Could you check a few things on this model? Use its own coordinates, in mm. A direction names the side the tool comes from. Give positions to 0.01 mm unless a question says otherwise; leave off trailing zeros. Write each loop counter-clockwise with the first axis right and the second up, starting at its lowest first coordinate (ties: lowest second). Pieces come first, ordered by that corner, then holes. Notation, with made-up numbers: (-20, 50) - (10, 50) arc R34 cw to (10, 85) - close; hole circle Ø9 at (84, 48). An arc over 180 degrees is marked (long way). Answer in a Markdown table with one row per item.
from build123d import *

# Parameters (mm, degrees)
SKETCH_1_R          = 1
SKETCH_1_R_2        = 1.5
EXTRUDE_1_DEPTH     = 4
SKETCH_2_W          = 10
SKETCH_2_H          = 4
SKETCH_2_W_2        = 4
CUT_EXTRUDE_3_DEPTH = 10


with BuildPart() as part:
    # Эскиз1 → Бобышка-Вытянуть1 (new body)
    with BuildSketch(Plane.XY):
        with BuildLine():
            Line((47, -12.5), (55, -12.5))
            Line((55, -12.5), (55, 12.5))
            Line((55, 12.5), (47, 12.5))
            Line((47, 12.5), (47, 10))
            Line((47, 10), (0, 10))
            ThreePointArc((0, 10), (-10, 0), (0, -10))
            Line((0, -10), (47, -10))
            Line((47, -10), (47, -12.5))
        make_face()
        with Locations((49, 10.5)):
            Circle(SKETCH_1_R, mode=Mode.SUBTRACT)
        with Locations(Location((49, -10.5, 0), (0, 0, 180))):
            Circle(SKETCH_1_R, mode=Mode.SUBTRACT)
        Circle(SKETCH_1_R_2, mode=Mode.SUBTRACT)
        with Locations((0, 7)):
            Circle(SKETCH_1_R_2, mode=Mode.SUBTRACT)
        with Locations((7, 0)):
            Circle(SKETCH_1_R_2, mode=Mode.SUBTRACT)
        with Locations((0, -7)):
            Circle(SKETCH_1_R_2, mode=Mode.SUBTRACT)
        with Locations((-7, 0)):
            Circle(SKETCH_1_R_2, mode=Mode.SUBTRACT)
    extrude(amount=EXTRUDE_1_DEPTH)

    # Эскиз2 → Вырез-Вытянуть3 (cut)
    with BuildSketch(Plane.XY.offset(4)):
        with Locations((30, 8)):
            Rectangle(SKETCH_2_W, SKETCH_2_H)
        with Locations((30, -8)):
            Rectangle(SKETCH_2_W, SKETCH_2_H)
        with Locations((22, 0)):
            Rectangle(SKETCH_2_W_2, SKETCH_2_H)
        Polygon((36, -2), (40, -2), (40, -18.487947924), (59.066234822, -18.487947924), (59.066234822, 17.495643995), (40, 17.495643995), (40, 2), (36, 2), align=None)
    extrude(amount=-CUT_EXTRUDE_3_DEPTH, mode=Mode.SUBTRACT)


solid = part.part
1) Will these pins go through, and if not, where does the flat tip stop? P1, Ø1.8, axis at x = 0, y = 0, coming from the +Z side; P2, Ø2, axis at y = -1.5, z = 1.5, coming from the -X side; P3, Ø2, axis at y = 0.5, z = 2, coming from the +X side; P4, Ø1.5, axis at x = -4, z = 2, coming from the +Y side.
Check values:
| item | result |
|---|---|
| P1 | passes through |
| P2 | stops at x = -9.99 |
| P3 | stops at x = 36 |
| P4 | stops at y = 9.46 |
2) Imagine slicing it at D-D (x = -7). List the corners of the cut face in (y, z) for me.
Check values:
| item | result |
|---|---|
| outline | (-7.14, 0) - (-1.5, 0) - (-1.5, 4) - (-7.14, 4) - close; (1.5, 0) - (7.14, 0) - (7.14, 4) - (1.5, 4) - close |
3) If I drill on line 1 (Y direction, x = 0, z = 0.85); line 2 (Y direction, x = 23.5, z = 0.5); line 3 (X direction, y = 6.25, z = 3.25), over which ranges is the centre line in solid material (lowest first)?
Check values:
| item | result |
|---|---|
| line 1 | y = -10 to -8.5, -5.5 to -1.5, 1.5 to 5.5, 8.5 to 10 |
| line 2 | y = -10 to -2, 2 to 10 |
| line 3 | x = -7.81 to -1.3, 1.3 to 25, 35 to 40 |
4) We'd pull the mould along Y, two halves only. Please class faces 4 (the face through (25, 8, 2)), 5 (the face through (30, -6, 2)), 6 (the face through (13, 10, 2)), 7 (the face through (36, 0, 2)): +Y half, -Y half, draft (parallel to the pull), parting line (faces both ways), or undercut.
Check values:
| item | result |
|---|---|
| face 4 | draft |
| face 5 | -Y half |
| face 6 | +Y half |
| face 7 | undercut |
5) On a 3-axis mill with a long thin cutter (end or side, diameter ignored), from which of +Z, -Z, +X, -X, +Y, -Y can I reach the whole of each face in a straight line? I mean faces 1 (the face through (22, -2, 2)), 2 (the face through (35, 8, 2)), 3 (the face through (38, 2, 2)). Say none if no direction works.
Check values:
| item | result |
|---|---|
| face 1 | +Z, -Z |
| face 2 | +Z, -Z, +Y |
| face 3 | +Z, -Z, +X |
6) Imagine slicing it at A-A (z = 0.75). List the corners of the cut face in (x, y) for me, then the cut area to 3 significant figures.
Check values:
| item | result |
|---|---|
| outline | (0, -10) - (25, -10) - (25, -6) - (35, -6) - (35, -10) - (40, -10) - (40, -2) - (36, -2) - (36, 2) - (40, 2) - (40, 10) - (35, 10) - (35, 6) - (25, 6) - (25, 10) - (0, 10) arc R10 ccw to start; hole circle Ø3 at (-7, 0); hole circle Ø3 at (0, -7); hole circle Ø3 at (0, 0); hole circle Ø3 at (0, 7); hole circle Ø3 at (7, 0); hole (20, -2) - (24, -2) - (24, 2) - (20, 2) - close |
| area | 810 mm2 |
7) Imagine slicing it at C-C (y = -8). List the corners of the cut face in (x, z) for me.
Check values:
| item | result |
|---|---|
| outline | (-6, 0) - (-1.12, 0) - (-1.12, 4) - (-6, 4) - close; (1.12, 0) - (25, 0) - (25, 4) - (1.12, 4) - close; (35, 0) - (40, 0) - (40, 4) - (35, 4) - close |
8) Imagine slicing it at B-B (y = 0). List the corners of the cut face in (x, z) for me, then the cut area to 3 significant figures.
Check values:
| item | result |
|---|---|
| outline | (-10, 0) - (-8.5, 0) - (-8.5, 4) - (-10, 4) - close; (-5.5, 0) - (-1.5, 0) - (-1.5, 4) - (-5.5, 4) - close; (1.5, 0) - (5.5, 0) - (5.5, 4) - (1.5, 4) - close; (8.5, 0) - (20, 0) - (20, 4) - (8.5, 4) - close; (24, 0) - (36, 0) - (36, 4) - (24, 4) - close |
| area | 132 mm2 |
